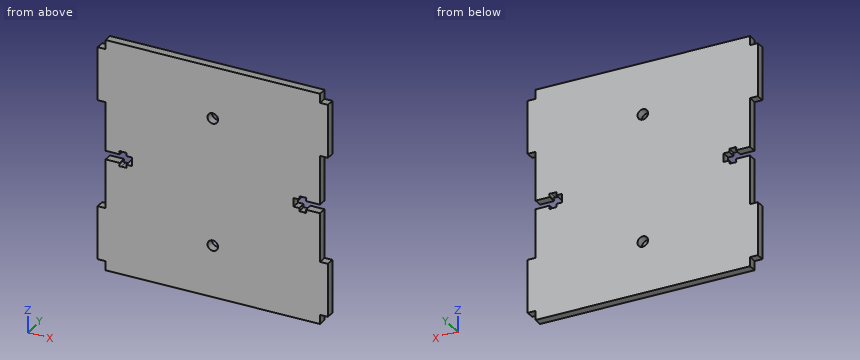
Autodesk Inventor part; units mm, degrees
ref_plane "YZ Plane" through (0, 0, 0) normal (1, 0, 0) x (0, 1, 0)
ref_plane "XZ Plane" through (0, 0, 0) normal (0, 1, 0) x (-1, 0, 0)
ref_plane "XY Plane" through (0, 0, 0) normal (0, 0, 1) x (1, 0, 0)
sketch "Sketch1" plane through (0, 0, 0) normal (0, 1, 0) x (-1, 0, 0)
  line L0 (38.2, 41.375) -> (0, 41.375)
  line L1 (0, -41.375) -> (38.2, -41.375)
  line L2 (38.2, -41.375) -> (38.2, -38.1)
  line L3 (38.2, 41.375) -> (-38.2, -41.375) construction
  line L4 (-38.2, 41.375) -> (38.2, -41.375) construction
  line L5 (38.2, -38.1) -> (41, -38.1)
  line L6 (41, -38.1) -> (41, -19.05)
  line L7 (41, 38.1) -> (38.2, 38.1)
  line L8 (41, -19.05) -> (38.2, -19.05)
  line L9 (41, 19.05) -> (38.2, 19.05)
  line L10 (0, -57.1711) -> (0, 53.4379)
  line L11 (38.2, -38.1) -> (38.2, -19.05) construction
  line L12 (38.2, -19.05) -> (38.2, -1.55)
  line L13 (38.2, 19.05) -> (38.2, 38.1) construction
  line L14 (38.2, 38.1) -> (38.2, 41.375)
  line L15 (41, 19.05) -> (41, 38.1)
  line L16 (41, -19.05) -> (41, 19.05) construction
  line L17 (43.0653, 0) -> (18.1238, 0)
  line L18 (38.2, 1.55) -> (33.2, 1.55)
  line L19 (33.2, 1.55) -> (33.2, 2.1343)
  line L20 (33.2, 2.7) -> (32.6343, 2.7) construction
  line L21 (30.8, 2.7) -> (30.8, 1.55)
  line L22 (30.8, 1.55) -> (28.8, 1.55)
  line L23 (28.8, 1.55) -> (28.8, 0)
  arc A0 (33.2, 2.1343) -> (32.6343, 2.7) centre (32.9172, 2.4172) ccw
  line L24 (33.2, 2.1343) -> (33.2, 2.7) construction
  line L25 (32.6343, 2.7) -> (30.8, 2.7)
  line L26 (38.2, -1.55) -> (33.2, -1.55)
  line L27 (33.2, -1.55) -> (33.2, -2.1343)
  line L28 (30.8, -2.7) -> (30.8, -1.55)
  line L29 (30.8, -1.55) -> (28.8, -1.55)
  line L30 (28.8, -1.55) -> (28.8, 0)
  arc A1 (32.6343, -2.7) -> (33.2, -2.1343) centre (32.9172, -2.4172) ccw
  line L31 (32.6343, -2.7) -> (30.8, -2.7)
  line L32 (38.2, -1.55) -> (38.2, 1.55) construction
  line L33 (38.2, 1.55) -> (38.2, 19.05)
  line L34 (-38.2, 41.375) -> (0, 41.375)
  line L35 (0, -41.375) -> (-38.2, -41.375)
  line L36 (-38.2, -41.375) -> (-38.2, -38.1)
  line L37 (-38.2, -38.1) -> (-41, -38.1)
  line L38 (-41, -38.1) -> (-41, -19.05)
  line L39 (-41, 38.1) -> (-38.2, 38.1)
  line L40 (-41, -19.05) -> (-38.2, -19.05)
  line L41 (-41, 19.05) -> (-38.2, 19.05)
  line L42 (-38.2, -19.05) -> (-38.2, -1.55)
  line L43 (-38.2, 38.1) -> (-38.2, 41.375)
  line L44 (-41, 19.05) -> (-41, 38.1)
  line L45 (-38.2, 1.55) -> (-33.2, 1.55)
  line L46 (-33.2, 1.55) -> (-33.2, 2.1343)
  line L47 (-30.8, 2.7) -> (-30.8, 1.55)
  line L48 (-30.8, 1.55) -> (-28.8, 1.55)
  line L49 (-28.8, 1.55) -> (-28.8, 0)
  arc A2 (-32.6343, 2.7) -> (-33.2, 2.1343) centre (-32.9172, 2.4172) ccw
  line L50 (-32.6343, 2.7) -> (-30.8, 2.7)
  line L51 (-38.2, -1.55) -> (-33.2, -1.55)
  line L52 (-33.2, -1.55) -> (-33.2, -2.1343)
  arc A3 (-33.2, -2.1343) -> (-32.6343, -2.7) centre (-32.9172, -2.4172) ccw
  line L53 (-30.8, -2.7) -> (-30.8, -1.55)
  line L54 (-30.8, -1.55) -> (-28.8, -1.55)
  line L55 (-28.8, -1.55) -> (-28.8, 0)
  line L56 (-38.2, 1.55) -> (-38.2, 19.05)
  line L57 (-32.6343, -2.7) -> (-30.8, -2.7)
  point P0 (0, 0)
  point P1 (0, 0)
  dimension "d0" = 76.4
  dimension "d2" = 76.2
  dimension "d3" = 2.8
  dimension "d4" = 19.05
  dimension "d5" = 82.75
  dimension "d6" = 3.1
  dimension "d7" = 5
  dimension "d8" = 0.4
  dimension "d9" = 2.4
  dimension "d10" = 5.4
  dimension "d11" = 2
extrude "Extrusion1" add sketch "Sketch1" along normal blind 3
sketch "Sketch2" plane through (0, 0, 0) normal (0, -1, 0) x (1, 0, 0)
  circle A0 centre (0, -22.86) radius 16 construction
  circle A1 centre (0, 22.86) radius 16 construction
  circle A2 centre (0, -22.86) radius 1.8844
  circle A3 centre (0, 22.86) radius 1.8844
  point P0 (0, 0)
  dimension "d14" = 32
  dimension "d15" = 22.86
  dimension "d16" = 22.86
  dimension "d17" = 3.7687
extrude "Extrusion2" cut sketch "Sketch2" against normal through all
properties part number "MountBase"
CAD build for the part. Positions are in the model's coordinates, mm. Round coordinates to 2 decimals unless told otherwise and drop trailing zeros. Write each loop counter-clockwise with the first axis right and the second up, starting at its lowest first coordinate (ties: lowest second). Pieces come first, ordered by that corner, then holes. Notation, with made-up numbers: M 88,50.25 L 143,50.25 A31 ccw 143,85.25 Z; hole C 61.25,-1.5 d4. An arc over 180 degrees is marked long. One line per question, with ' | ' between items.
1. Pin check, flat tips, straight feed: pin 1 Ø0.6 at (y, z) = (1.5, -2) entering from +X; pin 2 Ø2.5 at (x, z) = (0, -22.86) entering from +Y; pin 3 Ø0.9 at (y, z) = (1, 39.5) entering from -X; pin 4 Ø12 at (x, z) = (-6, -26.5) entering from -Y. Stop position of each tip, or through.
Working result:
pin 1: x = 38.2 | pin 2: through | pin 3: x = -38.2 | pin 4: y = 0
2. Probe L1, parallel to Z at x = 0, y = 0.7 (3 decimals); L2, parallel to Z at x = 29.5, y = 2.65 (3 decimals); L3, parallel to X at y = 2.05, z = 19. List the from-to ranges inside material, lowest first. Write a range as from..to.
Working result:
L1: -41.375..-24.744, -20.976..20.976, 24.744..41.375 | L2: -41.375..-1.55, 1.55..41.375 | L3: -38.2..38.2
3. Cut at C-C on y = 1.15. Count the separate pieces of the cut face and the enclosed holes in it, and give its area (3 significant figures).
Working result:
separate pieces: 1 | enclosed holes: 2 | area: 6,440 mm2
4. Cut at B-B on z = -22.86. Write the cut outline in (x, y).
Working result:
outline: M -41,0 L -1.88,0 L -1.88,3 L -41,3 Z; M 1.88,0 L 41,0 L 41,3 L 1.88,3 Z
5. Cut at A-A on x = 0. Write the cut outline in (y, z) (3 decimals).
Working result:
outline: M 0,-41.375 L 3,-41.375 L 3,-24.744 L 0,-24.744 Z; M 0,-20.976 L 3,-20.976 L 3,20.976 L 0,20.976 Z; M 0,24.744 L 3,24.744 L 3,41.375 L 0,41.375 Z
6. Cut at D-D on z = -7.5. Write the cut outline in (x, y).
Working result:
outline: M -38.2,0 L 38.2,0 L 38.2,3 L -38.2,3 Z
